Autodesk Inventor part; units mm, degrees
sketch "Esboço1" plane through (0, 0, 0) normal (0, 0, 1) x (1, 0, 0)
  circle A0 centre (0, 0) radius 6
  dimension "d0" = 12
extrude "Extrusão1" add sketch "Esboço1" along normal mid plane 100
sketch "Esboço2" plane through (0, 0, 50) normal (0, 0, 1) x (1, 0, 0)
  line L0 (5, 8.6603) -> (10, 0)
  line L1 (10, 0) -> (5, -8.6603)
  line L2 (5, -8.6603) -> (-5, -8.6603)
  line L3 (-5, -8.6603) -> (-10, 0)
  line L4 (-10, 0) -> (-5, 8.6603)
  line L5 (-5, 8.6603) -> (5, 8.6603)
  point P0 (0, 0)
  point P1 (0, 0)
  dimension "d3" = 10
extrude "Extrusão2" add sketch "Esboço2" along normal blind 5
thread "Rosca1"
chamfer "Chanfro1" distance 2 angle 45 1 edges at (-6, 0, 50)
chamfer "Chanfro2" distance 5 angle 45 1 edges at (-6, 0, -50)
properties part number "Sessao9__08_04_2025_0002_001" material "Ouro"
The model under review builds one solid part; all positions refer to its coordinate system, in mm. A direction names the side the tool comes from. Round coordinates to 2 decimals unless told otherwise and drop trailing zeros. Loops run counter-clockwise (first coordinate to the right, second up) from the corner with the lowest first, then second, coordinate; pieces in that order, holes last. Notation, with made-up numbers: (4, 3.25) - (45, 3.25) arc R23 ccw to (45, 33.25) - close; hole circle Ø4 at (21.5, -33). An arc over 180 degrees is marked (long way). Use CSV: the item, a comma, the result in double quotes.
(1) The part is to be moulded in two halves that separate along X. For faces 1 (the flat face through (0, -8.66, 52)), 2 (the flat face through (7.535, -4.27, 52.465)), 3 (the conical face through (0, -2, -49)), say which applies: pulls with the +X half, pulls with the -X half, needs draft (parallel to the pull), parting line crosses it, or undercut.
Working result:
face 1,"needs draft"
face 2,"pulls with the +X half"
face 3,"parting line crosses it"
(2) For line 1 (X direction, y = -0.25, z = -2); line 2 (X direction, y = -1.5, z = 32.5); line 3 (Y direction, x = 2, z = -26.5), list the stretches that pass through material, from the lowest coordinate up.
Working result:
line 1,"x = -5.99 to 5.99"
line 2,"x = -5.81 to 5.81"
line 3,"y = -5.66 to 5.66"
(3) Take a section at A-A, the plane x = 0. Give the boundary of the cut face in (y, z), plus the area to 3 significant figures.
Working result:
outline,"(-8.66, 50) - (-8, 50) - (-6, 48) - (-6, -45) - (-1, -50) - (1, -50) - (6, -45) - (6, 48) - (8, 50) - (8.66, 50) - (8.66, 55) - (-8.66, 55) - close"
area,"1,270 mm^2"
(4) Machinability: for faces 4 (the cylindrical face through (-6, 0, 1)), 5 (the flat face through (-7.535, 4.27, 52.465)), which of the approach directions +Z, -Z, +X, -X, +Y, -Y give a long, thin tool a straight path to every point of the face, cutting with its end or side? Answer none if there is none.
Working result:
face 4,"-Z"
face 5,"+Z, -Z, -X, +Y"
(5) Take a section at B-B, the plane z = 35. Give the boundary of the cut face in (x, y), plus the area to 3 significant figures.
Working result:
outline,"circle Ø12 at (0, 0)"
area,"113 mm^2"
(6) Clearance check with flat-ended pins moving along their axes: P1, Ø3, axis at x = 1.5, y = -2.5, coming from the -Z side; P2, Ø1, axis at x = -1.5, z = -29.5, coming from the +Y side; P3, Ø8, axis at y = -5.5, z = 9, coming from the -X side. State where each tip first meets the part, or that it passes through.
Working result:
P1,"stops at z = -49.58"
P2,"stops at y = 5.92"
P3,"stops at x = -5.81"
